Model file for the job. Use its own axes, mm. A direction names the side the tool comes from. Round coordinates to 2 decimals unless told otherwise and drop trailing zeros. Loops run counter-clockwise (first coordinate to the right, second up) from the corner with the lowest first, then second, coordinate; pieces in that order, holes last.
from build123d import *

# Parameters (mm, degrees)
ESQUISSE1_W          = 13.5
ESQUISSE1_H          = 35
ESQUISSE1_R          = 1.75
BOSS_EXTRU_1_DEPTH   = 2
BOSS_EXTRU_1_2_DEPTH = 2
ESQUISSE2_W          = 100
ESQUISSE2_H          = 35
ESQUISSE2_R          = 3
BOSS_EXTRU_2_DEPTH   = 4.5


with BuildPart() as part:
    # Esquisse1 → Boss.-Extru.1 (new body)
    with BuildSketch(Plane.XY):
        with Locations((-43.25, -17.5)):
            Rectangle(ESQUISSE1_W, ESQUISSE1_H)
        with Locations((-46.5, -7.5)):
            Circle(ESQUISSE1_R, mode=Mode.SUBTRACT)
        with Locations((-46.5, -27.5)):
            Circle(ESQUISSE1_R, mode=Mode.SUBTRACT)
    extrude(amount=BOSS_EXTRU_1_DEPTH)



with BuildPart() as body_2:
    # Esquisse1 → Boss.-Extru.1 2 (new body)
    with BuildSketch(Plane.XY):
        with Locations((43.25, -17.5)):
            Rectangle(ESQUISSE1_W, ESQUISSE1_H)
        with Locations(Location((46.5, -27.5, 0), (0, 0, 180))):
            Circle(ESQUISSE1_R, mode=Mode.SUBTRACT)
        with Locations(Location((46.5, -7.5, 0), (0, 0, 180))):
            Circle(ESQUISSE1_R, mode=Mode.SUBTRACT)
    extrude(amount=BOSS_EXTRU_1_2_DEPTH)


with BuildPart() as part_1:
    add(part.part)

    add(body_2.part)  # Boss.-Extru.2 merges body 2
    # Esquisse2 → Boss.-Extru.2 (add)
    with BuildSketch(Plane.XY.offset(2)):
        with Locations((0, -17.5)):
            Rectangle(ESQUISSE2_W, ESQUISSE2_H)
        with Locations((-46.5, -7.5)):
            Circle(ESQUISSE2_R, mode=Mode.SUBTRACT)
        with Locations((-46.5, -27.5)):
            Circle(ESQUISSE2_R, mode=Mode.SUBTRACT)
        with Locations((46.5, -7.5)):
            Circle(ESQUISSE2_R, mode=Mode.SUBTRACT)
        with Locations((46.5, -27.5)):
            Circle(ESQUISSE2_R, mode=Mode.SUBTRACT)
        with Locations((-26.5, -7.5)):
            Circle(ESQUISSE2_R, mode=Mode.SUBTRACT)
        with Locations((-26.5, -27.5)):
            Circle(ESQUISSE2_R, mode=Mode.SUBTRACT)
        with Locations(Location((26.5, -27.5, 0), (0, 0, 180))):
            Circle(ESQUISSE2_R, mode=Mode.SUBTRACT)
        with Locations(Location((26.5, -7.5, 0), (0, 0, 180))):
            Circle(ESQUISSE2_R, mode=Mode.SUBTRACT)
    extrude(amount=BOSS_EXTRU_2_DEPTH)


solid = part_1.part
Q1. Slice it at C-C on x = -26.5. Give the cut face in (y, z).
Q2. Probe line 1 (Y direction, x = 26.5, z = 5.35); line 2 (X direction, y = -27, z = 1.5); line 3 (Y direction, x = -46.5, z = 1.4). List the from-to ranges inside material, lowest first.
Q3. Flat gauge pins, fed straight in: P1, Ø5, axis at x = -46.5, y = -27.5, coming from the +Z side; P2, Ø3.5, axis at x = 26.5, y = -7.5, coming from the -Z side; P3, Ø10.5, axis at x = -2.5, y = -20.5, coming from the -Z side. Where does each tip first touch, or does it go through?
Q4. Pull direction Y, two halves, no side cores. Call faces 1 (the face through (-43, -17, 0)), 2 (the face through (-1, -35, 4)), 3 (the face through (-29.5, -7.4, 4.2)), 4 (the face through (-1, 0, 4)): pulls with the +Y half, pulls with the -Y half, needs draft (parallel to the pull), parting line crosses it, or undercut.
Q5. Slice it at D-D on y = -12. Give the cut face in (x, z), plus the area to 3 significant figures.
Q6. Slice it at A-A on z = 5. State how many separate pieces and enclosed holes the cut face has, plus the area to 3 significant figures.
Q7. Tool access for faces 5 (the face through (36.5, -18, 1)), 6 (the face through (43.5, -27.4, 4.2)), 7 (the face through (-1, -17, 6.5)): list every direction of +Z, -Z, +X, -X, +Y, -Y with a clear straight run to the whole face (end or side of a thin tool).
Reply:
1. outline: (-35, 2) - (-30.5, 2) - (-30.5, 6.5) - (-35, 6.5) - close; (-24.5, 2) - (-10.5, 2) - (-10.5, 6.5) - (-24.5, 6.5) - close; (-4.5, 2) - (0, 2) - (0, 6.5) - (-4.5, 6.5) - close
2. line 1: y = -35 to -30.5, -24.5 to -10.5, -4.5 to 0
2. line 2: x = -50 to -48.18, -44.82 to -36.5, 36.5 to 44.82, 48.18 to 50
2. line 3: y = -35 to -29.25, -25.75 to -9.25, -5.75 to 0
3. P1: stops at z = 2
3. P2: passes through
3. P3: stops at z = 2
4. face 1: needs draft
4. face 2: pulls with the -Y half
4. face 3: undercut
4. face 4: pulls with the +Y half
5. outline: (-50, 0) - (-36.5, 0) - (-36.5, 2) - (36.5, 2) - (36.5, 0) - (50, 0) - (50, 6.5) - (-50, 6.5) - close
5. area: 504 mm2
6. separate pieces: 1
6. enclosed holes: 8
6. area: 3,270 mm2
7. face 5: -Z, +Y, -Y
7. face 6: +Z
7. face 7: +Z, +X, -X, +Y, -Y
